from build123d import *

# Parameters (mm, degrees)
CUT_EXTRUDE1_DEPTH       = 44
FILLET1_R                = 1
CIRPATTERN1_COUNT        = 18
FILLET1_OF_CIRPATTERN1_R = 1
SKETCH4_R                = 4.125
CUT_EXTRUDE2_DEPTH       = 10


with BuildPart() as part:
    # Sketch1 → Revolve1 (revolve)
    with BuildSketch(Plane.XY):
        Polygon((0, 0), (-10, 0), (-10, 5), (-10, 12), (-10, 22), (0, 22), (0, 20), (0, 5), align=None)
    revolve(axis=Axis((0, 0, 0), (-1, 0, 0)))

    # Sketch2 → Cut-Extrude1 (cut)
    with BuildSketch(Plane(origin=(0, 0, 0), x_dir=(0, 0, -1), z_dir=(1, 0, 0))):
        Polygon((-2.5, 24), (2.5, 24), (1.5, 18), (-1.5, 18), align=None)
    cut_extrude1 = extrude(amount=-CUT_EXTRUDE1_DEPTH, mode=Mode.SUBTRACT)

    # Fillet1
    fillet1_edges = [part.edges().sort_by_distance(p)[0] for p in [
        (-5, 21.894776607, -2.149129435),
        (-5, 21.894776607, 2.149129435),
    ]]
    fillet(fillet1_edges, radius=FILLET1_R)

    # CirPattern1: Cut-Extrude1 ×18 about axis
    cirpattern1_axis = Axis((0, 0, 0), (1, 0, 0))
    for i in range(1, CIRPATTERN1_COUNT):
        add(cut_extrude1.rotate(cirpattern1_axis, i * 360 / CIRPATTERN1_COUNT), mode=Mode.SUBTRACT)

    # Fillet1 of CirPattern1
    fillet1_of_cirpattern1_edges = [part.edges().sort_by_distance(p)[0] for p in [
        (-5, 21.309405569, 5.468933563),
        (-5, 19.839314454, 9.507975704),
        (-5, 18.153805725, 12.427362459),
        (-5, 15.390938181, 15.720019781),
        (-5, 12.80858899, 17.886868035),
        (-5, 9.086187617, 20.035997469),
        (-5, 5.918467388, 21.188953343),
        (-5, 1.685508729, 21.935338163),
        (-5, -1.685508729, 21.935338163),
        (-5, -5.918467388, 21.188953343),
        (-5, -9.086187617, 20.035997469),
        (-5, -12.80858899, 17.886868035),
        (-5, -15.390938181, 15.720019781),
        (-5, -18.153805725, 12.427362459),
        (-5, -19.839314454, 9.507975704),
        (-5, -21.309405569, 5.468933563),
        (-5, -21.894776607, 2.149129435),
        (-5, -21.894776607, -2.149129435),
        (-5, -21.309405569, -5.468933563),
        (-5, -19.839314454, -9.507975704),
        (-5, -18.153805725, -12.427362459),
        (-5, -15.390938181, -15.720019781),
        (-5, -12.80858899, -17.886868035),
        (-5, -9.086187617, -20.035997469),
        (-5, -5.918467388, -21.188953343),
        (-5, -1.685508729, -21.935338163),
        (-5, 1.685508729, -21.935338163),
        (-5, 5.918467388, -21.188953343),
        (-5, 9.086187617, -20.035997469),
        (-5, 12.80858899, -17.886868035),
        (-5, 15.390938181, -15.720019781),
        (-5, 18.153805725, -12.427362459),
        (-5, 19.839314454, -9.507975704),
        (-5, 21.309405569, -5.468933563),
    ]]
    fillet(fillet1_of_cirpattern1_edges, radius=FILLET1_OF_CIRPATTERN1_R)

    # Sketch4 → Cut-Extrude2 (cut)
    with BuildSketch(Plane.ZY.offset(10)):
        Circle(SKETCH4_R)
    extrude(amount=-CUT_EXTRUDE2_DEPTH, mode=Mode.SUBTRACT)


solid = part.part
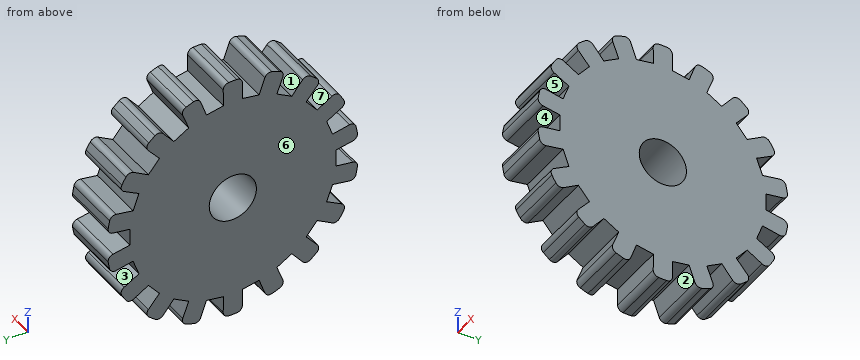
The listing builds one solid part. Answer for the finished solid, in the listing's coordinates (mm). Face numbers are marked on the shaded views. A direction names the side the tool comes from. Coordinates: 2 decimals unless noted, no trailing zeros. Write each loop counter-clockwise with the first axis right and the second up, starting at its lowest first coordinate (ties: lowest second). Pieces come first, ordered by that corner, then holes. Notation, with made-up numbers: M 67,-38.5 L 90,-38.5 A19 cw 90,-30.5 Z; hole C 34.25,-28.75 d9. An arc over 180 degrees is marked long. Use one line per item in the form item = value.
Item 1: The mould has two halves that part along Y. Classify the marked faces 5, 6 and 7: released by +Y, released by -Y, zero draft, split by the parting line, or undercut.
Model answer:
face_5 = released by -Y
face_6 = zero draft
face_7 = undercut
Item 2: Find section B-B, the plane z = 0. Give the vertices of the cut face in (x, y) (3 decimals), plus the area to 4 significant figures.
Model answer:
outline = M -10,-18 L 0,-18 L 0,-4.125 L -10,-4.125 Z; M -10,4.125 L 0,4.125 L 0,18 L -10,18 Z
area = 277.5 mm2
Item 3: Find the intervals of material crossed by probe 1 along Y at (x, z) = (-4.25, 0) (3 decimals); probe 2 along Y at (x, z) = (-4, 16); probe 3 along Z at (x, y) = (-5.5, 19), in increasing order.
Model answer:
probe_1 = -18 to -4.125, 4.125 to 18
probe_2 = -14.94 to -11.26, -8.29 to 8.29, 11.26 to 14.94
probe_3 = -11.09 to -9.03, -5.04 to -1.67, 1.67 to 5.04, 9.03 to 11.09
Item 4: Find section A-A, the plane y = 0. Give the vertices of the cut face in (x, z) (3 decimals), plus the area to 4 significant figures.
Model answer:
outline = M -10,-22 L 0,-22 L 0,-4.125 L -10,-4.125 Z; M -10,4.125 L 0,4.125 L 0,22 L -10,22 Z
area = 357.5 mm2
Item 5: For the marked faces 1, 2, 3 and 4, determine the directions among +Z, -Z, +X, -X, +Y, -Y from which every point of the face is accessible in a straight line to the end or side of a thin tool.
Model answer:
face_1 = +Z, +X, -X
face_2 = -Z, +X, -X
face_3 = +X, -X, +Y
face_4 = +X, -X, -Y
Item 6: Given P1, Ø3.5, axis at x = -6, z = -0.5, coming from the +Y side; P2, Ø0.9, axis at x = -6.5, z = -0.5, coming from the -Y side; P3, Ø2, axis at x = -3.5, y = 10, coming from the +Z side, each flat-ended and moving along its own axis, determine where each tip first touches the part or whether it passes through.
Model answer:
P1 = 21.47
P2 = -18
P3 = 15.69
Item 7: Find section C-C, the plane z = -14. Give the vertices of the cut face in (x, y).
Model answer:
outline = M -10,-13.92 L 0,-13.92 L 0,13.92 L -10,13.92 Z
